The figure shows three views and two pictorial views of one solid part (mm, origin at its lowest corner). Answer the questions. Coordinates: 2 decimals unless noted, no trailing zeros. Order: outer loops, then holes, each group sorted by start corner. A loop starts at its lowest first (then second) coordinate and runs counter-clockwise, first axis right, second up. Notation, with made-up numbers: (-17.5, -6) - (-3.5, -6) arc R30 ccw to (-3.5, 17) - close; hole circle Ø11 at (18, 7.5). An arc over 180 degrees is marked (long way). Use one line per item in the form item = value. Start each with the question number.
Item 1: Section C-C, the plane x = 134 is taken. Write down the section's boundary in (y, z).
Item 2: Section A-A, the plane z = 5 is taken. Write down the section's boundary in (x, y), and give its area (3 significant figures).
Item 3: Consider line 1 along X through (y, z) = (2.5, 4); line 2 along Y through (x, z) = (150.5, 5.5); line 3 along Y through (x, z) = (29, 6.5). Determine where each line is inside the solid, lowest interval first. Write a range as [from, to].
Item 4: Each of these flat-tipped pins is pushed along its axis until it touches: pin 1 Ø6 at (x, y) = (127.5, 8.5) entering from -Z; pin 2 Ø3 at (x, z) = (23.5, 2.5) entering from -Y. Where does it stop, or does it pass through?
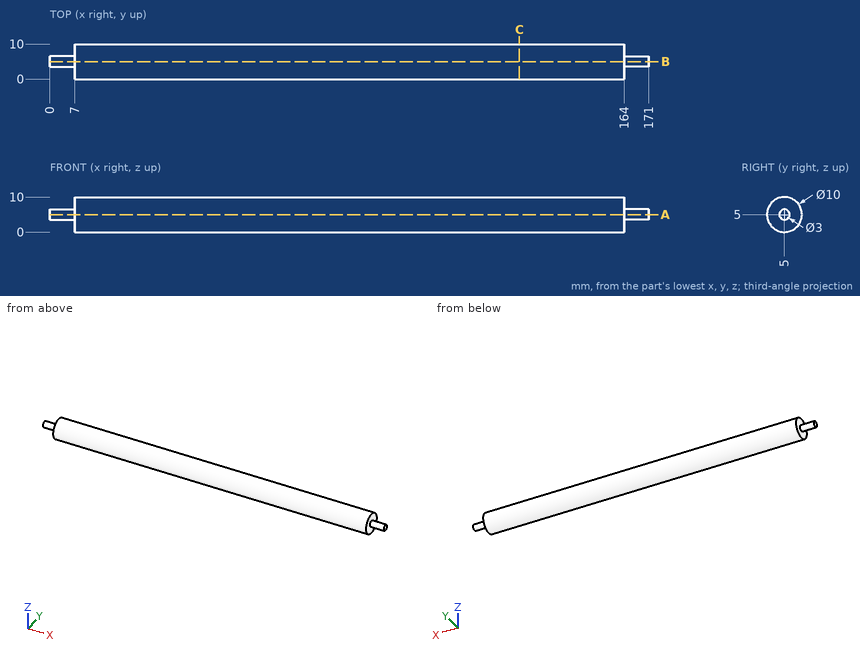
Response:
q1.outline = circle Ø10 at (5, 5)
q2.outline = (0, 3.5) - (7, 3.5) - (7, 0) - (164, 0) - (164, 3.5) - (171, 3.5) - (171, 6.5) - (164, 6.5) - (164, 10) - (7, 10) - (7, 6.5) - (0, 6.5) - close
q2.area = 1,610 mm2
q3.line_1 = [7, 164]
q3.line_2 = [0.03, 9.97]
q3.line_3 = [0.23, 9.77]
q4.pin_1 = 0.03
q4.pin_2 = 0.1
